Source: CAD feature listing. Evaluate the final solid. Frame: model axes, mm. A direction names the side the tool comes from. Give positions to 0.01 mm unless a question says otherwise; leave off trailing zeros. Answer as a JSON object with one key per item and string values. Group by question number.
```python
from build123d import *

# Parameters (mm, degrees)
F0_W      = 375
F0_H      = 375
F2_W      = 310
F2_H      = 310
F5_W      = 310
F5_H      = 310
F3_FACE_W = 310
F3_FACE_H = 310
F7_T      = 1
F14_R     = 4.5
F15_DEPTH = 345.4090421903
F16_R     = 4.5
F17_DEPTH = 345.4090421903


with BuildPart() as f3:
    # F0 (on Front) → F3 section 0
    with BuildSketch(Plane.XZ):
        Rectangle(F0_W, F0_H)
    # F2 (on offset) → F3 section 1
    with BuildSketch(Plane.XZ.offset(-20)):
        Rectangle(F2_W, F2_H)
    loft()

    # F5 (on offset) → F6 section 0
    with BuildSketch(Plane.XZ.offset(-36)):
        Rectangle(F5_W, F5_H)
    # F3_face (on face) → F6 section 1
    with BuildSketch(Plane(origin=(0, 20, 0), x_dir=(-1, 0, 0), z_dir=(0, 1, 0))):
        Rectangle(F3_FACE_W, F3_FACE_H)
    loft()

    # F7
    f7_openings = [f3.faces().sort_by_distance(p)[0] for p in [
        (0, 0, 0),
        (0, 36, 0),
    ]]
    offset(amount=F7_T, openings=f7_openings, kind=Kind.INTERSECTION)

    # F8 (on face) → F9 (revolve, cut)
    with BuildSketch(Plane(origin=(-156, 0, 0), x_dir=(0, -1, 0), z_dir=(-1, 0, 0))):
        with BuildLine():
            Line((-20.558795194, 146), (-20.558795194, 156))
            Line((-20.558795194, 156), (-36, 156))
            Line((-36, 156), (-36, 133.4152411143))
            ThreePointArc((-36, 133.4152411143), (-33.0658481949, 138.0710584905), (-27.6298630059, 138.9289321881))
            Line((-27.6298630059, 138.9289321881), (-20.558795194, 146))
        make_face()
    revolve(axis=Axis((-156, 28.279397597, 156), (0, 1, 0)), mode=Mode.SUBTRACT)

    # F8 (on face) → F10 (revolve, cut)
    with BuildSketch(Plane(origin=(-156, 0, 0), x_dir=(0, -1, 0), z_dir=(-1, 0, 0))):
        with BuildLine():
            Line((-36, -156), (-20.558795194, -156))
            Line((-20.558795194, -156), (-20.558795194, -146))
            Line((-20.558795194, -146), (-27.6298630059, -138.9289321881))
            ThreePointArc((-27.6298630059, -138.9289321881), (-33.0658481949, -138.0710584905), (-36, -133.4152411143))
            Line((-36, -133.4152411143), (-36, -156))
        make_face()
    revolve(axis=Axis((-156, 28.279397597, -156), (0, 1, 0)), mode=Mode.SUBTRACT)

    # F11 (on face) → F12 (revolve, cut)
    with BuildSketch(Plane.YZ.offset(156)):
        with BuildLine():
            Line((27.6298630059, -138.9289321881), (20.558795194, -146))
            Line((20.558795194, -146), (20.558795194, -156))
            Line((20.558795194, -156), (36, -156))
            Line((36, -156), (36, -133.4152411143))
            ThreePointArc((36, -133.4152411143), (33.0658481949, -138.0710584905), (27.6298630059, -138.9289321881))
        make_face()
    revolve(axis=Axis((156, 28.279397597, -156), (0, 1, 0)), mode=Mode.SUBTRACT)

    # F11 (on face) → F13 (revolve, cut)
    with BuildSketch(Plane.YZ.offset(156)):
        with BuildLine():
            Line((36, 156), (20.558795194, 156))
            Line((20.558795194, 156), (20.558795194, 146))
            Line((20.558795194, 146), (27.6298630059, 138.9289321881))
            ThreePointArc((27.6298630059, 138.9289321881), (33.0658481949, 138.0710584905), (36, 133.4152411143))
            Line((36, 133.4152411143), (36, 156))
        make_face()
    revolve(axis=Axis((156, 28.279397597, 156), (0, 1, 0)), mode=Mode.SUBTRACT)

    # F14 (on face) → F15 (cut, through all)
    with BuildSketch(Plane(origin=(0, 0, -156), x_dir=(1, 0, 0), z_dir=(0, 0, -1))):
        with Locations((-25, -28)):
            Circle(F14_R)
        with Locations((25, -28)):
            Circle(F14_R)
        with Locations((-87.5, -28)):
            Circle(F14_R)
        with Locations((87.5, -28)):
            Circle(F14_R)
    extrude(amount=-F15_DEPTH, mode=Mode.SUBTRACT)

    # F16 (on face) → F17 (cut, through all)
    with BuildSketch(Plane(origin=(-156, 0, 0), x_dir=(0, -1, 0), z_dir=(-1, 0, 0))):
        with Locations((-28, 25)):
            Circle(F16_R)
        with Locations((-28, 87.5)):
            Circle(F16_R)
        with Locations((-28, -25)):
            Circle(F16_R)
        with Locations((-28, -87.5)):
            Circle(F16_R)
    extrude(amount=-F17_DEPTH, mode=Mode.SUBTRACT)


solid = f3.part
```
(1) Section A-A, the plane x = 25. State how many separate pieces and enclosed holes the cut face has, plus the area to 3 significant figures.
(2) Pull-direction query (Y, two-part tool) for faces 1 (the flat face through (-2, 28, -155)), 2 (the cylindrical face through (155.49, 28.59, 91.96)), 3 (the flat face through (172.47, 10.423, -2.652)); classes: pulls with the +Y half, pulls with the -Y half, needs draft (parallel to the pull), parting line crosses it, or undercut.
(3) Ray query, L1, parallel to Z at x = -155.8, y = 28; L2, parallel to Z at x = -58, y = 28. Return the intervals inside material, ascending. Write a range as [from, to].
(4) Access query for faces 4 (the cylindrical face through (-155.51, 28.59, -83.04)), 5 (the flat face through (156, 28, -2)), 6 (the flat face through (-2, 28, -156)). Directions: +Z, -Z, +X, -X, +Y, -Y. A direction counts if a zero-diameter tool reaches every point of the face in a straight line with its end or side. Return the directions, or none.
(5) Contact query for flat-ended pins moving along their axis: pin 1 Ø5 at (x, y) = (-10, 27) entering from +Z; pin 2 Ø3 at (y, z) = (14.5, -41.5) entering from +X; pin 3 Ø1.5 at (y, z) = (19, -19) entering from +X; pin 4 Ø7 at (y, z) = (28, 25) entering from -X. Output: stop coordinate, or through.
Reported:
{
 "1": {"separate pieces": "4", "enclosed holes": "0", "area": "90.8 mm2"},
 "2": {"face 1": "needs draft", "face 2": "undercut", "face 3": "pulls with the +Y half"},
 "3": {"L1": "z = [-139.02, -92], [-83, -29.5], [-20.5, 20.5], [29.5, 83], [92, 139.02]", "L2": "z = [-156, -155], [155, 156]"},
 "4": {"face 4": "+X, -X", "face 5": "+Z, -Z, +X, +Y", "face 6": "-Z, +X, -X, +Y"},
 "5": {"pin 1": "stops at z = 156", "pin 2": "stops at x = 168.28", "pin 3": "stops at x = 159.75", "pin 4": "passes through"}
}
